Geometry: final body of the model. Coordinates: model frame, mm. A direction names the side the tool comes from. Give positions to 0.01 mm unless a question says otherwise; leave off trailing zeros. Write each loop counter-clockwise with the first axis right and the second up, starting at its lowest first coordinate (ties: lowest second). Pieces come first, ordered by that corner, then holes. Notation, with made-up numbers: (-28, 11) -> (26, 11) arc R25 ccw to (26, 34) -> close; hole circle Ø2 at (87, -37.75). An arc over 180 degrees is marked (long way). Use CSV: the item, a comma, the result in double quotes. Start each with the question number.
1) Section C-C (z = 7.5). Output: boundary loops of the cut face in (x, y).
2) Section B-B (z = 0). Output: boundary loops of the cut face in (x, y).
3) Material intervals for line 1 (Y direction, x = -9.7, z = 0); line 2 (X direction, y = 34.5, z = 2.5); line 3 (Z direction, x = -3.5, y = 12.5), sorted ascending. Write a range as [from, to].
4) Contact query for flat-ended pins moving along their axis: P1, Ø7, axis at y = 10, z = 0, coming from the -X side; P2, Ø12, axis at x = -1, z = 2.5, coming from the +Y side; P3, Ø1, axis at x = -7, y = 49.5, coming from the -Z side. Output: stop coordinate, or through.
5) Draft query along Y for faces 1 (the face through (0, 49, 9)), 2 (the face through (10, 10, 3)), 3 (the face through (2, 0, 10)), 4 (the face through (10.01, 87.07, 0.65)). Return one class per face: pulls with the +Y half, pulls with the -Y half, needs draft (parallel to the pull), parting line crosses it, or undercut.
6) Section A-A (y = 90). Output: boundary loops of the cut face in (x, z).
7) Section D-D (y = 76). Output: boundary loops of the cut face in (x, z), plus the area to 3 significant figures.
8) Set-up query: faces 5 (the face through (-9, 49, -1)), 6 (the face through (10, 49, -11)). Return all of +Z, -Z, +X, -X, +Y, -Y with unobstructed straight access to the full face (end or side cutting, diameter ignored); none if empty.
```python
from build123d import *

# Parameters (mm, degrees)
SALIENTE_EXTRUIR1_DEPTH = 100
CROQUIS2_R              = 3
CORTAR_EXTRUIR1_DEPTH   = 100
CROQUIS3_R              = 3
CORTAR_EXTRUIR2_DEPTH   = 103.980580694


with BuildPart() as part:
    # Croquis1 → Saliente-Extruir1 (new body)
    with BuildSketch(Plane(origin=(0, 0, 0), x_dir=(1, 0, 0), z_dir=(0, 1, 0))):
        Polygon((-9, 11), (-9, -9), (9, -9), (9, 11), (11, 11), (11, -11), (-11, -11), (-11, 11), align=None)
    extrude(amount=SALIENTE_EXTRUIR1_DEPTH)

    # Croquis2 → Cortar-Extruir1 (cut)
    with BuildSketch(Plane(origin=(11, 0, 0), x_dir=(0, 0, -1), z_dir=(1, 0, 0))):
        with Locations((0, 10)):
            Circle(CROQUIS2_R)
    extrude(amount=-CORTAR_EXTRUIR1_DEPTH, mode=Mode.SUBTRACT)

    # Croquis3 → Cortar-Extruir2 (cut, through all)
    with BuildSketch(Plane(origin=(11, 0, 0), x_dir=(0, 0, -1), z_dir=(1, 0, 0))):
        with Locations((0, 90)):
            Circle(CROQUIS3_R)
    extrude(amount=-CORTAR_EXTRUIR2_DEPTH, mode=Mode.SUBTRACT)


solid = part.part
```
Answers follow:
1,outline,"(-11, 0) -> (-9, 0) -> (-9, 100) -> (-11, 100) -> close; (9, 0) -> (11, 0) -> (11, 100) -> (9, 100) -> close"
2,outline,"(-11, 0) -> (-9, 0) -> (-9, 7) -> (-11, 7) -> close; (-11, 13) -> (-9, 13) -> (-9, 87) -> (-11, 87) -> close; (-11, 93) -> (-9, 93) -> (-9, 100) -> (-11, 100) -> close; (9, 0) -> (11, 0) -> (11, 7) -> (9, 7) -> close; (9, 13) -> (11, 13) -> (11, 87) -> (9, 87) -> close; (9, 93) -> (11, 93) -> (11, 100) -> (9, 100) -> close"
3,line 1,"y = [0, 7], [13, 87], [93, 100]"
3,line 2,"x = [-11, -9], [9, 11]"
3,line 3,"z = [9, 11]"
4,P1,"stops at x = -11"
4,P2,"passes through"
4,P3,"stops at z = 9"
5,face 1,"needs draft"
5,face 2,"undercut"
5,face 3,"pulls with the -Y half"
5,face 4,"undercut"
6,outline,"(-11, -11) -> (-9, -11) -> (-9, -3) -> (-11, -3) -> close; (-11, 3) -> (-9, 3) -> (-9, 9) -> (9, 9) -> (9, 3) -> (11, 3) -> (11, 11) -> (-11, 11) -> close; (9, -11) -> (11, -11) -> (11, -3) -> (9, -3) -> close"
7,outline,"(-11, -11) -> (-9, -11) -> (-9, 9) -> (9, 9) -> (9, -11) -> (11, -11) -> (11, 11) -> (-11, 11) -> close"
7,area,"124 mm^2"
8,face 5,"-Z, +Y, -Y"
8,face 6,"-Z, +X, -X, +Y, -Y"
